The model under review builds one solid part; all positions refer to its coordinate system, in mm. A direction names the side the tool comes from. Give positions to 0.01 mm unless a question says otherwise; leave off trailing zeros. Order: outer loops, then holes, each group sorted by start corner. A loop starts at its lowest first (then second) coordinate and runs counter-clockwise, first axis right, second up.
```python
from build123d import *

# Parameters (mm, degrees)
FLANGE_BASE1_DEPTH    = 3
FILETE1_R             = 11
FILETE2_R             = 11
CORTE_EXTRUS_O1_REACH = 43.113
ESBO_O2_R             = 5.25


# Sheet-metal steps are written as plain solids
with BuildPart() as part:
    # Esboço1 → Flange-base1 (new body)
    with BuildSketch(Plane.XY):
        with BuildLine():
            Line((-33, 6.5), (-8.874119675, 6.5))
            ThreePointArc((-8.874119675, 6.5), (-4.974937186, 9.810708435), (0, 11))
            ThreePointArc((0, 11), (4.974937186, 9.810708435), (8.874119675, 6.5))
            Line((8.874119675, 6.5), (33, 6.5))
            ThreePointArc((33, 6.5), (39.5, 0), (33, -6.5))
            Line((33, -6.5), (8.874119675, -6.5))
            ThreePointArc((8.874119675, -6.5), (4.974937186, -9.810708435), (0, -11))
            ThreePointArc((0, -11), (-4.974937186, -9.810708435), (-8.874119675, -6.5))
            Line((-8.874119675, -6.5), (-33, -6.5))
            ThreePointArc((-33, -6.5), (-39.5, 0), (-33, 6.5))
        make_face()
    extrude(amount=-FLANGE_BASE1_DEPTH)

    # Filete1
    filete1_edges = [part.edges().sort_by_distance(p)[0] for p in [
        (-8.874119675, 6.5, -1.5),
    ]]
    fillet(filete1_edges, radius=FILETE1_R)

    # Filete2
    filete2_edges = [part.edges().sort_by_distance(p)[0] for p in [
        (8.874119675, -6.5, -1.5),
        (-8.874119675, -6.5, -1.5),
        (8.874119675, 6.5, -1.5),
    ]]
    fillet(filete2_edges, radius=FILETE2_R)

    # Esboço2 → Corte-extrusão1 (cut, up to next)
    with BuildSketch(Plane(origin=(0, 0, -3), x_dir=(-1, 0, 0), z_dir=(0, 0, -1)), mode=Mode.PRIVATE) as corte_extrus_o1_sk1:
        Circle(ESBO_O2_R)
    corte_extrus_o1_tool1 = extrude(corte_extrus_o1_sk1.sketch, amount=-CORTE_EXTRUS_O1_REACH, mode=Mode.PRIVATE) & part.part
    add(corte_extrus_o1_tool1.solids().sort_by_distance((0, 0, -3))[0], mode=Mode.SUBTRACT)


solid = part.part
```
Item 1: Draft analysis for pull direction Y (two halves, no side actions). For faces 1 (the flat face through (23, 6.5, -1)), 2 (the flat face through (-23, -6.5, -1)), 3 (the cylindrical face through (-39.5, -0.1, -1.5)), 4 (the cylindrical face through (-5, 1.6, -1.5)), state which applies: released by +Y, released by -Y, zero draft, split by the parting line, or undercut.
Values found:
face 1: released by +Y
face 2: released by -Y
face 3: split by the parting line
face 4: undercut
Item 2: For faces 5 (the flat face through (-23, 6.5, -1)), 6 (the flat face through (1, -7, 0)), 7 (the flat face through (23, -6.5, -1)), list the 3-axis set-ups (+Z, -Z, +X, -X, +Y, -Y) from which the entire face can be reached by the end or side of a thin tool; tool diameter is ignored.
Values found:
face 5: +Z, -Z, -X, +Y
face 6: +Z, +X, -X, +Y, -Y
face 7: +Z, -Z, +X, -Y
Item 3: Take a section at B-B (y = 0). Give the boundary of the cut face in (x, z).
Values found:
outline: (-39.5, -3) - (-5.25, -3) - (-5.25, 0) - (-39.5, 0) - close; (5.25, -3) - (39.5, -3) - (39.5, 0) - (5.25, 0) - close
Item 4: Take a section at A-A (z = -1.85). Give the boundary of the cut face in (x, y), and give its area (3 significant figures).
Values found:
outline: (-33, -6.5) - (-13.33, -6.5) arc R11 cw to (-6.67, -8.75) arc R11 ccw to (6.67, -8.75) arc R11 cw to (13.33, -6.5) - (33, -6.5) arc R6.5 ccw to (33, 6.5) - (13.33, 6.5) arc R11 cw to (6.67, 8.75) arc R11 ccw to (-6.67, 8.75) arc R11 cw to (-13.33, 6.5) - (-33, 6.5) arc R6.5 ccw to start; hole circle Ø10.5 at (0, 0)
area: 1,020 mm2
Item 5: Take a section at C-C (x = -1.5). Give the boundary of the cut face in (y, z), and give its area (3 significant figures).
Values found:
outline: (-10.9, -3) - (-5.03, -3) - (-5.03, 0) - (-10.9, 0) - close; (5.03, -3) - (10.9, -3) - (10.9, 0) - (5.03, 0) - close
area: 35.2 mm2
Item 6: For line 1 (Y direction, x = 29, z = -0.85); line 2 (X direction, y = 2, z = -0.55); line 3 (X direction, y = 2.25, z = -1.55), list the stretches that pass through material, from the lowest coordinate up.
Values found:
line 1: y = -6.5 to 6.5
line 2: x = -39.18 to -4.85, 4.85 to 39.18
line 3: x = -39.1 to -4.74, 4.74 to 39.1
Item 7: Take a section at D-D (x = 10). Give the boundary of the cut face in (y, z).
Values found:
outline: (-7.02, -3) - (7.02, -3) - (7.02, 0) - (-7.02, 0) - close
Item 8: Clearance check with flat-ended pins moving along their axes: pin 1 Ø1.5 at (x, z) = (25.5, -2) entering from +Y; pin 2 Ø9.5 at (x, y) = (0, 0) entering from +Z; pin 3 Ø1.5 at (x, z) = (-27, -2) entering from -Y; pin 4 Ø1 at (y, z) = (-1.5, -1) entering from +X. State where each tip first meets the part, or that it passes through.
Values found:
pin 1: stops at y = 6.5
pin 2: passes through
pin 3: stops at y = -6.5
pin 4: stops at x = 39.42
